Could you check a few things on this model? Use its own coordinates, in mm. A direction names the side the tool comes from. Coordinates: 2 decimals unless noted, no trailing zeros. Loops run counter-clockwise (first coordinate to the right, second up) from the corner with the lowest first, then second, coordinate; pieces in that order, holes last. Notation, with made-up numbers: M 18.25,62 L 75.25,62 A27 ccw 75.25,86 Z; hole C 88.25,-29.5 d2. An arc over 180 degrees is marked long. Use one line per item in the form item = value. Start each with the question number.
```python
from build123d import *

# Parameters (mm, degrees)
PAD_DEPTH    = 5
POCKET_DEPTH = 5
CHAMFER_SIZE = 1
FILLET_R     = 1


with BuildPart() as part:
    # Sketch → Pad (new body)
    with BuildSketch(Plane.XY):
        with BuildLine():
            Line((0, 15), (0, 0))
            Line((0, 0), (15, 0))
            Line((15, 0), (30, 3))
            ThreePointArc((28, -6.38736), (34.799024, -2.929176), (30, 3))
            Line((28, -6.38736), (22.436801, -7.5))
            ThreePointArc((22.436801, -7.5), (38.399434, -6.141839), (30, 7.5))
            ThreePointArc((30, 7.5), (38.399434, 21.141839), (22.436801, 22.5))
            Line((22.436801, 22.5), (28, 21.38736))
            ThreePointArc((30, 12), (34.799024, 17.929176), (28, 21.38736))
            Line((15, 15), (30, 12))
            Line((0, 15), (15, 15))
        make_face()
    extrude(amount=PAD_DEPTH)

    # Sketch001 (on Face13 of Pad) → Pocket (cut)
    with BuildSketch(Plane.XY.offset(5)):
        with BuildLine():
            ThreePointArc((7, 12.5), (6, 13.5), (5, 12.5))
            Line((5, 12.5), (5, 2.5))
            ThreePointArc((5, 2.5), (6, 1.5), (7, 2.5))
            Line((7, 12.5), (7, 2.5))
        make_face()
        with BuildLine():
            ThreePointArc((12, 12.5), (11, 13.5), (10, 12.5))
            Line((10, 12.5), (10, 2.5))
            ThreePointArc((10, 2.5), (11, 1.5), (12, 2.5))
            Line((12, 12.5), (12, 2.5))
        make_face()
    extrude(amount=-POCKET_DEPTH, mode=Mode.SUBTRACT)

    # Chamfer
    chamfer_edges = [part.edges().sort_by_distance(p)[0] for p in [
        (7, 7.5, 5),
        (10, 7.5, 5),
        (7, 7.5, 0),
        (10, 7.5, 0),
        (22.436801, 22.5, 2.5),
        (22.436801, -7.5, 2.5),
    ]]
    chamfer(chamfer_edges, length=CHAMFER_SIZE)

    # Fillet
    fillet_edges = [part.edges().sort_by_distance(p)[0] for p in [
        (0, 15, 2.5),
        (0, 0, 2.5),
    ]]
    fillet(fillet_edges, radius=FILLET_R)


solid = part.part
```
Item 1: I want a section at B-B (z = 2.05). Write out the boundary of the cut face in (x, y).
Item 2: Thinking about a two-plate mould opening in Y: for faces 5 (the flat face through (0, 8, 2)), 6 (the cylindrical face through (38.714, 20.449, 2.465)), 7 (the flat face through (8, 15, 2)), which applies, pulls with the +Y half, pulls with the -Y half, needs draft (parallel to the pull), parting line crosses it, or undercut?
Item 3: I want a section at C-C (x = 33). Write out the boundary of the cut face in (y, z), plus the area to 3 significant figures.
Item 4: I'm going to push flat-ended pins straight in: P1, Ø1.5, axis at y = 7, z = 2.5, coming from the +X side; P2, Ø1.5, axis at x = 9, z = 2, coming from the -Y side; P3, Ø3, axis at x = 27.5, z = 0.5, coming from the -Y side. Where does each tip first touch, or does it pass through?
Item 5: Please list where these lines run through material, in increasing order: line 1 along X through (y, z) = (5, 4.6); line 2 along Y through (x, z) = (26, 3.7); line 3 along X through (y, z) = (6, 4.5).
Item 6: For faces 1 (the conical face through (6, 1.2, 4.3)), 2 (the flat face through (12, 8, 3)), 3 (the flat face through (12.5, 7.4, 0.5)), 4 (the flat face through (23.243, 22.794, 2.465)), which set-ups out of +Z, -Z, +X, -X, +Y, -Y let a thin tool reach every point of the face, with its end or its side?
Item 7: I want a section at A-A (x = 11). Write out the boundary of the cut face in (y, z).
Item 8: I want a section at D-D (x = 24.5). Write out the boundary of the cut face in (y, z), plus the area to 3 significant figures.
Worked answers:
q1.outline = M 0,1 A1 ccw 1,0 L 15,0 L 30,3 A4.91 cw long 28,-6.39 L 23.42,-7.3 L 23.07,-8.27 A9.41 ccw long 30,7.5 A9.41 ccw long 23.07,23.27 L 23.42,22.3 L 28,21.39 A4.91 cw long 30,12 L 15,15 L 1,15 A1 ccw 0,14 Z; hole M 5,2.5 A1 ccw 7,2.5 L 7,12.5 A1 ccw 5,12.5 Z; hole M 10,2.5 A1 ccw 12,2.5 L 12,12.5 A1 ccw 10,12.5 Z
q2.face_5 = needs draft
q2.face_6 = undercut
q2.face_7 = pulls with the +Y half
q3.outline = M -10.82,0 L -5.79,0 L -5.79,5 L -10.82,5 Z; M 1.98,0 L 7.01,0 L 7.01,5 L 1.98,5 Z; M 7.99,0 L 13.02,0 L 13.02,5 L 7.99,5 Z; M 20.79,0 L 25.82,0 L 25.82,5 L 20.79,5 Z
q3.area = 101 mm²
q4.P1 = 34.69
q4.P2 = 0
q4.P3 = -11.26
q5.line_1 = 0 to 4.4, 7.6 to 9.4, 12.6 to 36.39
q5.line_2 = -10.42 to -6.79, 2.2 to 12.8, 21.79 to 25.42
q5.line_3 = 0 to 4.5, 7.5 to 9.5, 12.5 to 35.1
q6.face_1 = +Z
q6.face_2 = +Z, -Z
q6.face_3 = -Z
q6.face_4 = +Z, -Z, -X
q7.outline = M 0,0 L 0.5,0 L 1.5,1 L 1.5,4 L 0.5,5 L 0,5 Z; M 13.5,1 L 14.5,0 L 15,0 L 15,5 L 14.5,5 L 13.5,4 Z
q8.outline = M -9.54,0 L -7.09,0 L -7.09,5 L -9.54,5 Z; M 1.9,0 L 13.1,0 L 13.1,5 L 1.9,5 Z; M 22.09,0 L 24.54,0 L 24.54,5 L 22.09,5 Z
q8.area = 80.5 mm²
